from build123d import *

# Parameters (mm, degrees)
F1_DEPTH = 304.8
F2_W     = 63.5
F2_H     = 57.15
F3_DEPTH = 6.35
F5_DEPTH = 6.35


with BuildPart() as f1:
    # F0 (on Front) → F1 (new body)
    with BuildSketch(Plane.XZ):
        Polygon((0, 38.1), (0, 0), (6.35, 0), (6.35, 101.6), (0, 101.6), (0, 44.45), (-63.5, 44.45), (-63.5, 38.1), align=None)
    extrude(amount=F1_DEPTH)

    # F2 (on face) → F3 (cut, through all)
    with BuildSketch(Plane.YZ.offset(6.35)):
        with Locations((-273.05, 73.025)):
            Rectangle(F2_W, F2_H)
        with Locations((-31.75, 73.025)):
            Rectangle(F2_W, F2_H)
        with BuildLine():
            Line((-168.275, 69.85), (-168.275, 82.55))
            ThreePointArc((-168.275, 82.55), (-177.8, 92.075), (-187.325, 82.55))
            Line((-187.325, 82.55), (-187.325, 69.85))
            ThreePointArc((-187.325, 69.85), (-177.8, 60.325), (-168.275, 69.85))
        make_face()
        with BuildLine():
            ThreePointArc((-117.475, 82.55), (-127, 92.075), (-136.525, 82.55))
            Line((-136.525, 82.55), (-136.525, 69.85))
            ThreePointArc((-136.525, 69.85), (-127, 60.325), (-117.475, 69.85))
            Line((-117.475, 69.85), (-117.475, 82.55))
        make_face()
    extrude(amount=-F3_DEPTH, mode=Mode.SUBTRACT)

    # F4 (on face) → F5 (cut, through all)
    with BuildSketch(Plane.XY.offset(44.45)):
        with BuildLine():
            Line((-25.4, -279.4), (-25.4, -228.6))
            ThreePointArc((-25.4, -228.6), (-34.925, -219.075), (-44.45, -228.6))
            Line((-44.45, -228.6), (-44.45, -279.4))
            ThreePointArc((-44.45, -279.4), (-34.925, -288.925), (-25.4, -279.4))
        make_face()
        with BuildLine():
            ThreePointArc((-44.45, -76.2), (-34.925, -85.725), (-25.4, -76.2))
            Line((-25.4, -76.2), (-25.4, -25.4))
            ThreePointArc((-25.4, -25.4), (-34.925, -15.875), (-44.45, -25.4))
            Line((-44.45, -25.4), (-44.45, -76.2))
        make_face()
    extrude(amount=-F5_DEPTH, mode=Mode.SUBTRACT)


solid = f1.part
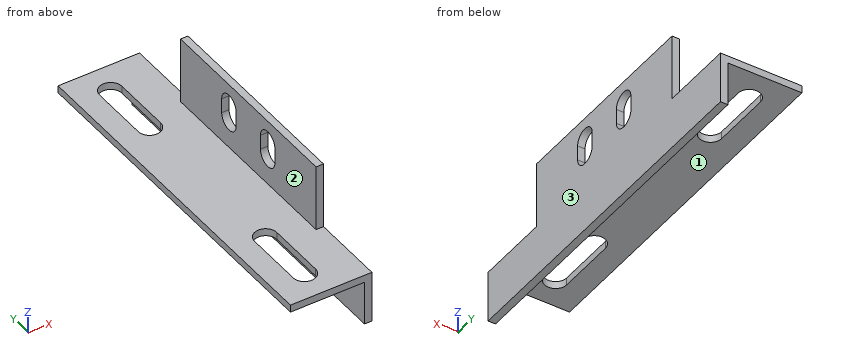
Can you work these out from the model? Positions are in its coordinate system, mm. Face numbers are marked on the shaded views. A direction names the side the tool comes from. Round coordinates to 2 decimals unless told otherwise and drop trailing zeros. Loops run counter-clockwise (first coordinate to the right, second up) from the corner with the lowest first, then second, coordinate; pieces in that order, holes last. Notation, with made-up numbers: (71, 78.25) - (113, 78.25) arc R11 cw to (113, 92.25) - close; hole circle Ø3 at (-37, 64.5). An arc over 180 degrees is marked (long way). Write item = value, one per line. Start each with the question number.
(1) If we section it at C-C (y = -177.8): Please give me the cut outline in (x, z) (3 decimals), and give its area (3 significant figures).
(2) For P1, Ø1.9, axis at x = 4.5, z = 76, coming from the -Y side; P2, Ø5, axis at x = 3, z = 73, coming from the +Y side; P3, Ø12, axis at y = -117, z = 71, coming from the -X side; P4, Ø12, axis at y = -49, z = 36, coming from the -X side, each with a flat end and sliding along its axis, tell me the tip position at first contact or that it passes through.
(3) If we section it at D-D (x = -8): Please give me the cut outline in (y, z), and give its area (3 significant figures).
(4) If we section it at A-A (y = -32.5): Please give me the cut outline in (x, z).
(5) If we section it at B-B (z = 41.5): Please give me the cut outline in (x, y) (3 decimals).
(6) For the marked faces 1, 2 and 3, which set-ups out of +Z, -Z, +X, -X, +Y, -Y let a thin tool reach every point of the face, with its end or its side?
(7) If I drill on probe 1 along Y at (x, z) = (2.5, 77.5) (3 decimals); probe 2 along Z at (x, y) = (-48.5, -113); probe 3 along X at (y, z) = (-174, 60), over which ranges is the centre line in solid material (lowest first)? Write a range as [from, to].
Ans:
q1.outline = (-63.5, 38.1) - (0, 38.1) - (0, 0) - (6.35, 0) - (6.35, 60.325) - (0, 60.325) - (0, 44.45) - (-63.5, 44.45) - close; (0, 92.075) - (6.35, 92.075) - (6.35, 101.6) - (0, 101.6) - close
q1.area = 847 mm²
q2.P1 = -241.3
q2.P2 = -63.5
q2.P3 = 0
q2.P4 = -63.5
q3.outline = (-304.8, 38.1) - (0, 38.1) - (0, 44.45) - (-304.8, 44.45) - close
q3.area = 1,940 mm²
q4.outline = (-63.5, 38.1) - (-44.45, 38.1) - (-44.45, 44.45) - (-63.5, 44.45) - close; (-25.4, 38.1) - (0, 38.1) - (0, 0) - (6.35, 0) - (6.35, 44.45) - (-25.4, 44.45) - close
q5.outline = (-63.5, -304.8) - (6.35, -304.8) - (6.35, 0) - (-63.5, 0) - close; hole (-44.45, -279.4) arc R9.525 ccw to (-25.4, -279.4) - (-25.4, -228.6) arc R9.525 ccw to (-44.45, -228.6) - close; hole (-44.45, -76.2) arc R9.525 ccw to (-25.4, -76.2) - (-25.4, -25.4) arc R9.525 ccw to (-44.45, -25.4) - close
q6.face_1 = -Z, -X, +Y, -Y
q6.face_2 = +Z, -X, +Y, -Y
q6.face_3 = +Z, -Z, +X, +Y, -Y
q7.probe_1 = [-241.3, -187.325], [-168.275, -136.525], [-117.475, -63.5]
q7.probe_2 = [38.1, 44.45]
q7.probe_3 = [0, 6.35]
